Geometry check sheet. Reference: the model listing, model coordinates, mm. Give positions to 0.01 mm unless a question says otherwise; leave off trailing zeros. Write each loop counter-clockwise with the first axis right and the second up, starting at its lowest first coordinate (ties: lowest second). Pieces come first, ordered by that corner, then holes. Notation, with made-up numbers: (74, 22.25) - (84, 22.25) arc R16 cw to (84, 46.25) - close; hole circle Ø10 at (69, -24.5). An arc over 180 degrees is marked (long way). Use a Markdown table: item, result.
Autodesk Inventor part; units mm, degrees
ref_plane "YZ Plane" through (0, 0, 0) normal (1, 0, 0) x (0, 1, 0)
ref_plane "XZ Plane" through (0, 0, 0) normal (0, 1, 0) x (-1, 0, 0)
ref_plane "XY Plane" through (0, 0, 0) normal (0, 0, 1) x (1, 0, 0)
sketch "Sketch1" plane through (0, 0, 0) normal (0, 1, 0) x (-1, 0, 0)
  line L0 (0, 0) -> (0, -3)
  line L1 (-250, -38) -> (-250, -78)
  line L2 (0, 0) -> (-20, 0)
  line L3 (-50, 0) -> (-50, -3)
  line L4 (-50, 0) -> (-70, 0)
  line L5 (-70, 0) -> (-70, -3)
  line L6 (-100, 0) -> (-100, -3)
  line L7 (-100, 0) -> (-120, 0)
  line L8 (-120, 0) -> (-120, -3)
  line L9 (-150, 0) -> (-150, -3)
  line L10 (-150, 0) -> (-170, 0)
  line L11 (-170, 0) -> (-170, -3)
  line L12 (-200, 0) -> (-200, -3)
  line L13 (-200, 0) -> (-220, 0)
  line L14 (-220, 0) -> (-220, -3)
  line L15 (-20, 0) -> (-20, -3)
  line L16 (-250, -58) -> (-250, -78)
  line L17 (-250, -78) -> (-247, -78)
  line L18 (-247, -78) -> (-247, -113)
  line L19 (-250, -58) -> (-250, -38)
  line L20 (-250, -38) -> (-247, -38)
  line L21 (-247, -38) -> (-247, -3)
  line L22 (-220, -3) -> (-247, -3)
  line L23 (-170, -3) -> (-200, -3)
  line L24 (-120, -3) -> (-150, -3)
  line L25 (-20, -3) -> (-50, -3)
  line L26 (-70, -3) -> (-100, -3)
  line L27 (0, -116) -> (0, -113)
  line L28 (0, -116) -> (-20, -116)
  line L29 (-50, -116) -> (-50, -113)
  line L30 (-50, -116) -> (-70, -116)
  line L31 (-70, -116) -> (-70, -113)
  line L32 (-100, -116) -> (-100, -113)
  line L33 (-100, -116) -> (-120, -116)
  line L34 (-120, -116) -> (-120, -113)
  line L35 (-150, -116) -> (-150, -113)
  line L36 (-150, -116) -> (-170, -116)
  line L37 (-170, -116) -> (-170, -113)
  line L38 (-200, -116) -> (-200, -113)
  line L39 (-200, -116) -> (-220, -116)
  line L40 (-220, -116) -> (-220, -113)
  line L41 (-20, -116) -> (-20, -113)
  line L42 (-3, -58) -> (-3, -78)
  line L43 (-3, -78) -> (0, -78)
  line L44 (-3, -58) -> (-3, -38)
  line L45 (-3, -38) -> (0, -38)
  line L46 (0, -113) -> (0, -78)
  line L47 (0, -38) -> (0, -3)
  line L48 (-50, -113) -> (-20, -113)
  line L49 (-100, -113) -> (-70, -113)
  line L50 (-150, -113) -> (-120, -113)
  line L51 (-247, -113) -> (-220, -113)
  line L52 (-200, -113) -> (-170, -113)
  dimension "d2" = 110
  dimension "d3" = 20
  dimension "d4" = 20
  dimension "d5" = 20
  dimension "d7" = 20
  dimension "d8" = 20
  dimension "d9" = 20
  dimension "d10" = 3
  dimension "d11" = 20
  dimension "d12" = 3
  dimension "d13" = 250
  dimension "d14" = 30
  dimension "d15" = 30
  dimension "d16" = 30
  dimension "d17" = 30
extrude "Extrusion1" add sketch "Sketch1" along normal blind 3
properties part number "latGenerico"
1) Section check A-A on x = 45. Record the boundary of the cut face in (y, z), then the cut area to 3 significant figures.
Working result:
| item | result |
|---|---|
| outline | (0, -113) - (3, -113) - (3, -3) - (0, -3) - close |
| area | 330 mm² |
2) Material ranges on L1, parallel to X at y = 0.15, z = -58; L2, parallel to X at y = 0.45, z = -94.5; L3, parallel to Z at x = 89, y = 0.85, recorded low to high. Write a range as from..to.
Working result:
| item | result |
|---|---|
| L1 | x = 3..250 |
| L2 | x = 0..247 |
| L3 | z = -113..-3 |
3) Depth check by flat-ended pin: P1, Ø1.5, axis at y = 1, z = -114.5, coming from the +X side; P2, Ø1.5, axis at y = 2, z = -23, coming from the +X side; P3, Ø0.9, axis at x = 239, y = 1.5, coming from the -Z side; P4, Ø0.9, axis at y = 1, z = -114, coming from the -X side. Enter the tip coordinate at first touch or a pass-through.
Working result:
| item | result |
|---|---|
| P1 | stops at x = 220 |
| P2 | stops at x = 247 |
| P3 | stops at z = -113 |
| P4 | stops at x = 0 |
